from build123d import *

# Parameters (mm, degrees)
SKETCH_R       = 3.5
PAD_DEPTH      = 2.5
PAD_DEPTH_BACK = 2.5
FILLET_R       = 1
FILLET001_R    = 1


with BuildPart() as part:
    # Sketch → Pad (new body, two sides)
    with BuildSketch(Plane.XZ) as pad_sk:
        Circle(SKETCH_R)
    extrude(amount=PAD_DEPTH)
    extrude(pad_sk.sketch, amount=-PAD_DEPTH_BACK)

    # Fillet
    fillet_edges = [part.edges().sort_by_distance(p)[0] for p in [
        (-3.5, -2.5, 0),
    ]]
    fillet(fillet_edges, radius=FILLET_R)

    # Fillet001
    fillet001_edges = [part.edges().sort_by_distance(p)[0] for p in [
        (-3.5, 2.5, 0),
    ]]
    fillet(fillet001_edges, radius=FILLET001_R)

    # Sketch001 → Revolution (revolve)
    with BuildSketch(Plane.XZ):
        with BuildLine():
            Line((0, -2.5), (2.4, -2.5))
            ThreePointArc((2.4, -2.5), (1.604465, -3.362015), (1.319973, -4.5))
            Line((0, -4.5), (1.319973, -4.5))
            Line((0, -2.5), (0, -4.5))
        make_face()
    revolve(axis=Axis((0, 0, 0), (0, 0, 1)))


solid = part.part
Build history of the part. All positions in model axes, mm. Give positions to 0.01 mm unless a question says otherwise; leave off trailing zeros. Loops run counter-clockwise (first coordinate to the right, second up) from the corner with the lowest first, then second, coordinate; pieces in that order, holes last. Notation, with made-up numbers: (-21.75, 14.25) -> (24.25, 14.25) arc R35 cw to (24.25, 47.25) -> close; hole circle Ø10 at (-24.5, 88.5). An arc over 180 degrees is marked (long way). Answer in a Markdown table with one row per item.
Item 1: Probe line 1 along Z through (x, y) = (-0.75, 1.95); line 2 along Z through (x, y) = (1, -0.75); line 3 along X through (y, z) = (-1.9, -1.5). List the from-to ranges inside material, lowest first. Write a range as [from, to].
Findings below:
| item | result |
|---|---|
| line 1 | z = [-3.31, 3.31] |
| line 2 | z = [-4.5, 3.35] |
| line 3 | x = [-3.07, 3.07] |
Item 2: Slice it at C-C on y = -1.95. Write the cut outline in (x, z).
Findings below:
| item | result |
|---|---|
| outline | circle Ø6.79 at (0, 0) |
Item 3: Slice it at B-B on z = 0. Write the cut outline in (x, y).
Findings below:
| item | result |
|---|---|
| outline | (-3.5, -1.5) arc R1 ccw to (-2.5, -2.5) -> (2.5, -2.5) arc R1 ccw to (3.5, -1.5) -> (3.5, 1.5) arc R1 ccw to (2.5, 2.5) -> (-2.5, 2.5) arc R1 ccw to (-3.5, 1.5) -> close |
Item 4: Slice it at D-D on z = -4. Write the cut outline in (x, y).
Findings below:
| item | result |
|---|---|
| outline | circle Ø2.74 at (0, 0) |
Item 5: Flat gauge pins, fed straight in: P1, Ø1.5, axis at y = -1, z = 2.5, coming from the +X side; P2, Ø2, axis at x = 2, y = 2, coming from the -Z side; P3, Ø4, axis at x = 2, z = 2, coming from the +Y side. Where does each tip first touch, or does it go through?
Findings below:
| item | result |
|---|---|
| P1 | stops at x = 3.03 |
| P2 | stops at z = -3.32 |
| P3 | stops at y = 2.5 |
Item 6: Slice it at A-A on x = 0. Write the cut outline in (y, z).
Findings below:
| item | result |
|---|---|
| outline | (-2.5, -2.5) arc R1 ccw to (-1.54, -3.5) arc R2.37 cw to (-1.32, -4.5) -> (1.32, -4.5) arc R2.37 cw to (1.54, -3.5) arc R1 ccw to (2.5, -2.5) -> (2.5, 2.5) arc R1 ccw to (1.5, 3.5) -> (-1.5, 3.5) arc R1 ccw to (-2.5, 2.5) -> close |
